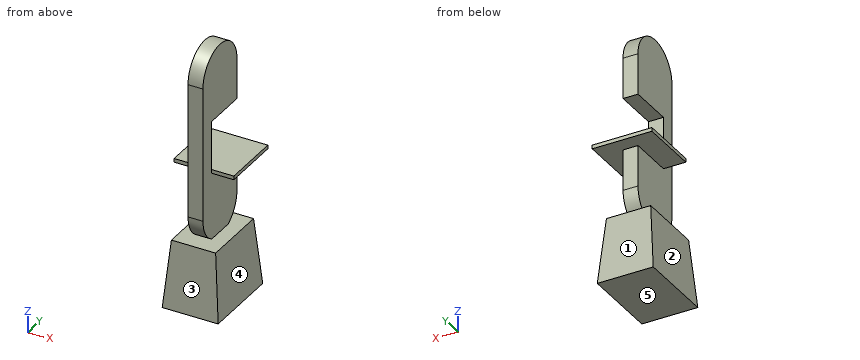
```python
from build123d import *

# Parameters (mm, degrees)
F0_W     = 381
F0_H     = 533.4
F1_DEPTH = 457.2
F1_TAPER = 5
F3_DEPTH = 50.8
F4_W     = 406.4
F4_H     = 406.4
F5_DEPTH = 25.4


with BuildPart() as f1:
    # F0 (on Top) → F1 (new body)
    with BuildSketch(Plane.XY):
        with Locations((0, 266.7)):
            Rectangle(F0_W, F0_H)
    extrude(amount=F1_DEPTH, taper=F1_TAPER)

    # F2 (on Right) → F3 (join, symmetric)
    with BuildSketch(Plane.YZ):
        with BuildLine():
            Line((63.5, 1549.4), (63.5, 635))
            ThreePointArc((63.5, 635), (266.7, 431.8), (469.9, 635))
            Line((469.9, 635), (469.9, 914.4))
            Line((469.9, 914.4), (165.1, 914.4))
            Line((165.1, 914.4), (165.1, 1270))
            Line((165.1, 1270), (469.9, 1270))
            Line((469.9, 1270), (469.9, 1549.4))
            ThreePointArc((469.9, 1549.4), (266.7, 1752.6), (63.5, 1549.4))
        make_face()
    extrude(amount=F3_DEPTH, both=True)

    # F4 (on face) → F5 (join)
    with BuildSketch(Plane.XY.offset(914.4)):
        with Locations((0, 368.3)):
            Rectangle(F4_W, F4_H)
    extrude(amount=F5_DEPTH)


solid = f1.part
```
Build history of the part. All positions in model axes, mm. Face numbers are marked on the shaded views. A direction names the side the tool comes from. Round coordinates to 2 decimals unless told otherwise and drop trailing zeros. Write each loop counter-clockwise with the first axis right and the second up, starting at its lowest first coordinate (ties: lowest second). Pieces come first, ordered by that corner, then holes.
1) Band-saw the part on B-B, the plane y = 289. List the corners of the cut face in (x, z), and give its area (3 significant figures).
2) Band-saw the part on C-C, the plane x = -11. List the corners of the cut face in (y, z).
3) 3-axis set-ups, long thin cutter, end or side, ignore diameter. For the marked faces 1 and 2: which of +Z, -Z, +X, -X, +Y, -Y reach the whole face in a straight line?
4) Mould opens along Z. For the marked faces 3, 4 and 5 say: +Z half, -Z half, draft (parallel to the pull), parting line (faces both ways), or undercut.
5) Band-saw the part on A-A, the plane x = -93. List the corners of the cut face in (y, z), and give its area (3 significant figures).
6) Pin check, flat tips, straight feed: pin 1 (12 mm diameter, centred on y = 108.5, z = 750, fed in from +X); pin 2 (5 mm diameter, centred on y = 445.5, z = 312.5, fed in from -X); pin 3 (2 mm diameter, centred on x = 12.5, z = 1055.5, fed in from +Y). Stop position of each tip, or through.
7) Band-saw the part on D-D, the plane z = 1062.5. List the corners of the cut face in (x, y), and give its area (3 significant figures).
8) Drill centre lines: probe 1 along Z at (x, y) = (79, 370); probe 2 along Z at (x, y) = (39, 431); probe 3 along Z at (x, y) = (88, 121). Where is each one in solid material? Low to high.
Ans:
1. outline: (-203.2, 914.4) - (-50.8, 914.4) - (-50.8, 457.2) - (-150.5, 457.2) - (-190.5, 0) - (190.5, 0) - (150.5, 457.2) - (50.8, 457.2) - (50.8, 914.4) - (203.2, 914.4) - (203.2, 939.8) - (-203.2, 939.8) - close; (-50.8, 1270) - (50.8, 1270) - (50.8, 1751.37) - (-50.8, 1751.37) - close
1. area: 262,000 mm2
2. outline: (0, 0) - (533.4, 0) - (493.4, 457.2) - (365.07, 457.2) arc R203.2 ccw to (469.9, 635) - (469.9, 914.4) - (571.5, 914.4) - (571.5, 939.8) - (165.1, 939.8) - (165.1, 1270) - (469.9, 1270) - (469.9, 1549.4) arc R203.2 ccw to (63.5, 1549.4) - (63.5, 635) arc R203.2 ccw to (168.33, 457.2) - (40, 457.2) - close
3. face 1: +X, -X, +Y
3. face 2: -X, +Y, -Y
4. face 3: +Z half
4. face 4: undercut
4. face 5: -Z half
5. outline: (0, 0) - (533.4, 0) - (493.4, 457.2) - (40, 457.2) - close; (165.1, 914.4) - (571.5, 914.4) - (571.5, 939.8) - (165.1, 939.8) - close
5. area: 236,000 mm2
6. pin 1: stops at x = 50.8
6. pin 2: stops at x = -163.38
6. pin 3: stops at y = 165.1
7. outline: (-50.8, 63.5) - (50.8, 63.5) - (50.8, 165.1) - (-50.8, 165.1) - close
7. area: 10,300 mm2
8. probe 1: z = 0 to 457.2, 914.4 to 939.8
8. probe 2: z = 0 to 457.2, 515.44 to 939.8, 1270 to 1668.96
8. probe 3: z = 0 to 457.2
